Geometry check sheet. Reference: the model listing, model coordinates, mm. A direction names the side the tool comes from. Give positions to 0.01 mm unless a question says otherwise; leave off trailing zeros. Order: outer loops, then holes, each group sorted by start corner. A loop starts at its lowest first (then second) coordinate and runs counter-clockwise, first axis right, second up. Notation, with made-up numbers: M 42,42.25 L 92,42.25 A18 cw 92,63.25 Z; hole C 53,27 d7. An arc over 180 degrees is marked long. Answer as CSV lines item,"result".
from build123d import *

# Parameters (mm, degrees)
F0_R     = 2.875
F1_DEPTH = 1.75
F2_DEPTH = 18
F0_R_2   = 1.75
F3_DEPTH = 5
F4_W     = 4
F4_H     = 9
F5_DEPTH = 25


with BuildPart() as f1:
    # F0 (on Front) → F1 (new body)
    with BuildSketch(Plane.XZ):
        with BuildLine():
            ThreePointArc((-13, 33), (-15.12132, 32.12132), (-16, 30))
            Line((-16, 30), (-16, -30))
            ThreePointArc((-16, -30), (-15.12132, -32.12132), (-13, -33))
            Line((-13, -33), (13, -33))
            ThreePointArc((13, -33), (15.12132, -32.12132), (16, -30))
            Line((16, -30), (16, 30))
            ThreePointArc((16, 30), (15.12132, 32.12132), (13, 33))
            Line((13, 33), (-13, 33))
        make_face()
        with Locations((-11.5, -29)):
            Circle(F0_R, mode=Mode.SUBTRACT)
        with Locations((11.5, -29)):
            Circle(F0_R, mode=Mode.SUBTRACT)
        with Locations((-11.5, 29)):
            Circle(F0_R, mode=Mode.SUBTRACT)
        with Locations((11.5, 29)):
            Circle(F0_R, mode=Mode.SUBTRACT)
    extrude(amount=F1_DEPTH)

    # F0 (on Front) → F2 (join)
    with BuildSketch(Plane.XZ):
        with BuildLine():
            Line((13, 34.75), (-13, 34.75))
            ThreePointArc((-13, 34.75), (-16.358757, 33.358757), (-17.75, 30))
            Line((-17.75, 30), (-17.75, -30))
            ThreePointArc((-17.75, -30), (-16.358757, -33.358757), (-13, -34.75))
            Line((-13, -34.75), (13, -34.75))
            ThreePointArc((13, -34.75), (16.358757, -33.358757), (17.75, -30))
            Line((17.75, -30), (17.75, 30))
            ThreePointArc((17.75, 30), (16.358757, 33.358757), (13, 34.75))
        make_face()
        with BuildLine():
            Line((-16, -30), (-16, 30))
            ThreePointArc((-16, 30), (-15.12132, 32.12132), (-13, 33))
            Line((-13, 33), (13, 33))
            ThreePointArc((13, 33), (15.12132, 32.12132), (16, 30))
            Line((16, 30), (16, -30))
            ThreePointArc((16, -30), (15.12132, -32.12132), (13, -33))
            Line((13, -33), (-13, -33))
            ThreePointArc((-13, -33), (-15.12132, -32.12132), (-16, -30))
        make_face(mode=Mode.SUBTRACT)
    extrude(amount=F2_DEPTH)

    # F0 (on Front) → F3 (join)
    with BuildSketch(Plane.XZ):
        with Locations((-11.5, 29)):
            Circle(F0_R)
        with Locations((-11.5, 29)):
            Circle(F0_R_2, mode=Mode.SUBTRACT)
        with Locations((11.5, 29)):
            Circle(F0_R)
        with Locations((11.5, 29)):
            Circle(F0_R_2, mode=Mode.SUBTRACT)
        with Locations((11.5, -29)):
            Circle(F0_R)
        with Locations((11.5, -29)):
            Circle(F0_R_2, mode=Mode.SUBTRACT)
        with Locations((-11.5, -29)):
            Circle(F0_R)
        with Locations((-11.5, -29)):
            Circle(F0_R_2, mode=Mode.SUBTRACT)
    extrude(amount=F3_DEPTH)

    # F4 (on face) → F5 (cut)
    with BuildSketch(Plane.YZ.offset(17.75)):
        with Locations((-3.6589, 24.661605)):
            Rectangle(F4_W, F4_H)
    extrude(amount=-F5_DEPTH, mode=Mode.SUBTRACT)


solid = f1.part
(1) Tool access check on faces 5 (the face through (0, 0, 0)), 6 (the face through (-13.62, -3.35, -27.06)). Record the directions out of +Z, -Z, +X, -X, +Y, -Y that give a thin tool (end or side, any length) a straight path to the whole face; none if there is none.
The answers:
face 5,"+Z, -Z, +X, -X, +Y"
face 6,"-Y"
(2) Section check B-B on x = -11.5. Enter the section's corners in (y, z) (3 decimals).
The answers:
outline,"M -18,-34.75 L 0,-34.75 L 0,-30.75 L -5,-30.75 L -5,-31.875 L -1.75,-31.875 L -1.75,-33 L -18,-33 Z; M -18,33 L -1.75,33 L -1.75,31.875 L -5,31.875 L -5,30.75 L 0,30.75 L 0,34.75 L -18,34.75 Z; M -5,-27.25 L 0,-27.25 L 0,27.25 L -5,27.25 L -5,26.125 L -1.75,26.125 L -1.75,-26.125 L -5,-26.125 Z"
(3) Draft check along Z on faces 1 (the face through (-16.395, -8.874, -33.322)), 2 (the face through (15.1, -9.76, 32.14)), 3 (the face through (11.272, -1.909, 30.735)), 4 (the face through (-16.322, -8.874, 33.395)). Enter one of: +Z half, -Z half, draft (parallel to the pull), parting line (faces both ways), or undercut.
The answers:
face 1,"-Z half"
face 2,"undercut"
face 3,"undercut"
face 4,"+Z half"
(4) Material ranges on line 1 (Z direction, x = 11.5, y = -3.9) (3 decimals); line 2 (X direction, y = -16.5, z = -15.5); line 3 (Z direction, x = 0, y = -7.25), recorded low to high.
The answers:
line 1,"z = -34.75 to -33, -31.875 to -30.75, -27.25 to -26.125, 30.75 to 31.875, 33 to 34.75"
line 2,"x = -17.75 to -16, 16 to 17.75"
line 3,"z = -34.75 to -33, 33 to 34.75"
(5) Section check C-C on z = -29. Enter the section's corners in (x, y) (3 decimals).
The answers:
outline,"M -17.75,-18 L -16,-18 L -16,-1.75 L -14.375,-1.75 L -14.375,-5 L -13.25,-5 L -13.25,0 L -17.75,0 Z; M -9.75,-5 L -8.625,-5 L -8.625,-1.75 L 8.625,-1.75 L 8.625,-5 L 9.75,-5 L 9.75,0 L -9.75,0 Z; M 13.25,-5 L 14.375,-5 L 14.375,-1.75 L 16,-1.75 L 16,-18 L 17.75,-18 L 17.75,0 L 13.25,0 Z"
(6) Section check A-A on z = 21. Enter the section's corners in (x, y).
The answers:
outline,"M -17.75,-18 L -16,-18 L -16,-1.75 L -7.25,-1.75 L -7.25,-1.66 L 17.75,-1.66 L 17.75,0 L -17.75,0 Z; M 16,-18 L 17.75,-18 L 17.75,-5.66 L 16,-5.66 Z"
(7) Section check D-D on y = -13.25. Enter the section's corners in (x, z), then the cut area to 3 significant figures.
The answers:
outline,"M -17.75,-30 A4.75 ccw -13,-34.75 L 13,-34.75 A4.75 ccw 17.75,-30 L 17.75,30 A4.75 ccw 13,34.75 L -13,34.75 A4.75 ccw -17.75,30 Z; hole M -16,-30 A3 ccw -13,-33 L 13,-33 A3 ccw 16,-30 L 16,30 A3 ccw 13,33 L -13,33 A3 ccw -16,30 Z"
area,"344 mm2"
(8) Gauge pin test, flat ends, axial feed: P1, Ø4, axis at x = 11.5, z = 29, coming from the -Y side; P2, Ø1.2, axis at x = 16, y = -3.5, coming from the -Z side; P3, Ø7, axis at x = 8, z = 25, coming from the -Y side. Record the tip position at first contact, or that the pin passes through.
The answers:
P1,"stops at y = -5"
P2,"stops at z = -34.1"
P3,"stops at y = -1.66"
